Check sheet for the modelled part. Datum: model origin and axes. Units: mm. A direction names the side the tool comes from. Round coordinates to 2 decimals unless told otherwise and drop trailing zeros. Write each loop counter-clockwise with the first axis right and the second up, starting at its lowest first coordinate (ties: lowest second). Pieces come first, ordered by that corner, then holes.
Item 1: Release check for a two-part mould opening along Y. For faces 1 (the flat face through (-26, -13, 2)), 2 (the flat face through (-22, -13, 0.99)), 3 (the flat face through (-25, -35.09, 9)) record: +Y half, -Y half, draft (parallel to the pull), parting line (faces both ways), or undercut.
Item 2: Cross-section at B-B on x = -19. Enter the section's corners in (y, z).
Item 3: Cross-section at C-C on z = 18.5. Enter the section's corners in (x, y).
Item 4: Tool access check on faces 4 (the cylindrical face through (-19.49, 3.689, 3.287)), 5 (the cylindrical face through (-13.079, -2.82, 5.062)), 6 (the cylindrical face through (-19.438, -22.617, 3.561)), 7 (the flat face through (-9.914, -30, 10)), 8 (the cylindrical face through (-9.023, -30.055, 6.325)). Record the directions out of +Z, -Z, +X, -X, +Y, -Y that give a thin tool (end or side, any length) a straight path to the whole face; none if there is none.
Item 5: Cross-section at D-D on y = -1.5. Enter the section's corners in (x, z).
Item 6: Material ranges on line 1 (Y direction, x = -32, z = 17.25); line 2 (Y direction, x = -18.9, z = 6); line 3 (X direction, y = 1.5, z = 2.5), recorded low to high.
Item 7: Cross-section at A-A on y = 3. Enter the section's corners in (x, z), plus the area to 3 significant figures.
Item 8: Go/stop test with flat-tipped pins: pin 1 Ø1.6 at (y, z) = (2.5, 5.5) entering from -X; pin 2 Ø10 at (y, z) = (-30, 13.5) entering from +X; pin 3 Ø5 at (y, z) = (2.41, 6) entering from -X; pin 4 Ø8.5 at (x, y) = (-27.5, -15) entering from +Z. Record where each tip stops, or that it passes through.
from build123d import *

# Parameters (mm, degrees)
CROQUIS1_W               = 25
CROQUIS1_H               = 44
SALIENTE_EXTRUIR1_DEPTH  = 20
CROQUIS2_W               = 11.3
CROQUIS2_H               = 40.4
CORTAR_EXTRUIR1_DEPTH    = 18
CROQUIS3_W               = 10.7
CROQUIS3_H               = 44
CORTAR_EXTRUIR2_DEPTH    = 12
CORTAR_EXTRUIR3_START    = -25
CROQUIS4_R               = 1.6
CORTAR_EXTRUIR3_DEPTH    = 25
CROQUIS5_R               = 3
CORTAR_EXTRUIR4_DEPTH    = 17
CROQUIS7_W               = 10.7
CROQUIS7_H               = 2.131966011
SALIENTE_EXTRUIR2_DEPTH  = 12
CROQUIS9_W               = 11.3
CROQUIS9_H               = 12.16552506
SALIENTE_EXTRUIR3_DEPTH  = 2
SALIENTE_EXTRUIR4_DEPTH  = 2
CORTAR_EXTRUIR10_START   = -25
CROQUIS12_W              = 0.99
CROQUIS12_H              = 44
CORTAR_EXTRUIR10_DEPTH   = 25
CROQUIS13_W              = 8
CROQUIS13_H              = 44
CORTAR_EXTRUIR11_DEPTH   = 11.7
SALIENTE_EXTRUIR5_DEPTH  = 11.7
CROQUIS15_W              = 10.763613753
CROQUIS15_H              = 40.736067978
CORTAR_EXTRUIR12_DEPTH   = 4
CROQUIS16_R              = 1.5
SALIENTE_EXTRUIR6_DEPTH  = 1.2
CORTAR_EXTRUIR13_START   = -44
CORTAR_EXTRUIR13_DEPTH   = 44
CROQUIS18_W              = 0.936386247
CROQUIS18_H              = 40.568033989
CORTAR_EXTRUIR14_DEPTH   = 4
SALIENTE_EXTRUIR7_START  = -9.2
SALIENTE_EXTRUIR7_DEPTH  = 9.2
SALIENTE_EXTRUIR8_START  = -12.9
CROQUIS20_W              = 4
CROQUIS20_H              = 0.236067978
CROQUIS20_H_2            = 0.25
SALIENTE_EXTRUIR8_DEPTH  = 12.9
CROQUIS21_W              = 4
CROQUIS21_H              = 6.401046148
CROQUIS21_H_2            = 6.387114126
SALIENTE_EXTRUIR9_DEPTH  = 1.5
SALIENTE_EXTRUIR10_DEPTH = 0.4


with BuildPart() as part:
    # Croquis1 → Saliente-Extruir1 (new body)
    with BuildSketch(Plane.XY):
        with Locations((-22.114132301, -13.090425532)):
            Rectangle(CROQUIS1_W, CROQUIS1_H)
    extrude(amount=SALIENTE_EXTRUIR1_DEPTH)

    # Croquis2 → Cortar-Extruir1 (cut)
    with BuildSketch(Plane.XY.offset(20)):
        with Locations((-26.964132301, -13.090425532)):
            Rectangle(CROQUIS2_W, CROQUIS2_H)
    extrude(amount=-CORTAR_EXTRUIR1_DEPTH, mode=Mode.SUBTRACT)

    # Croquis3 → Cortar-Extruir2 (cut)
    with BuildSketch(Plane.XY.offset(20)):
        with Locations((-14.964132301, -13.090425532)):
            Rectangle(CROQUIS3_W, CROQUIS3_H)
    extrude(amount=-CORTAR_EXTRUIR2_DEPTH, mode=Mode.SUBTRACT)

    # Croquis4 → Cortar-Extruir3 (cut)
    with BuildSketch(Plane.ZY.offset(34.614132301).offset(CORTAR_EXTRUIR3_START)):
        with Locations((6, 2.409574468)):
            Circle(CROQUIS4_R)
        with Locations((6, -28.590425532)):
            Circle(CROQUIS4_R)
        with BuildLine():
            Line((20, 5.909574468), (20, -32.090425532))
            ThreePointArc((20, -32.090425532), (1, -13.090425532), (20, 5.909574468))
        make_face()
    extrude(amount=CORTAR_EXTRUIR3_DEPTH, mode=Mode.SUBTRACT)

    # Croquis5 → Cortar-Extruir4 (cut)
    with BuildSketch(Plane.ZY.offset(34.614132301)):
        with Locations((6, 2.409574468)):
            Circle(CROQUIS5_R)
        with Locations((6, -28.590425532)):
            Circle(CROQUIS5_R)
    extrude(amount=-CORTAR_EXTRUIR4_DEPTH, mode=Mode.SUBTRACT)

    # Croquis7 → Saliente-Extruir2 (add)
    with BuildSketch(Plane.XY.offset(8)):
        with Locations((-14.964132301, -34.024442527)):
            Rectangle(CROQUIS7_W, CROQUIS7_H)
        with Locations((-14.964132301, 7.843591463)):
            Rectangle(CROQUIS7_W, CROQUIS7_H)
    extrude(amount=SALIENTE_EXTRUIR2_DEPTH)

    # Croquis9 → Saliente-Extruir3 (add)
    with BuildSketch(Plane.XY.offset(2)):
        with Locations((-26.964132301, -13.090425532)):
            Rectangle(CROQUIS9_W, CROQUIS9_H)
    extrude(amount=-SALIENTE_EXTRUIR3_DEPTH)

    # Croquis11 → Saliente-Extruir4 (add)
    with BuildSketch(Plane.ZY.offset(32.614132301)):
        with BuildLine():
            Line((2, -7.007663002), (2, -19.173188062))
            ThreePointArc((2, -19.173188062), (1, -13.090425532), (2, -7.007663002))
        make_face()
    extrude(amount=SALIENTE_EXTRUIR4_DEPTH)

    # Croquis12 → Cortar-Extruir10 (cut)
    with BuildSketch(Plane.ZY.offset(34.614132301).offset(CORTAR_EXTRUIR10_START)):
        with Locations((0.495, -13.090425532)):
            Rectangle(CROQUIS12_W, CROQUIS12_H)
    extrude(amount=CORTAR_EXTRUIR10_DEPTH, mode=Mode.SUBTRACT)

    # Croquis13 → Cortar-Extruir11 (cut)
    with BuildSketch(Plane(origin=(-9.614132301, 0, 0), x_dir=(0, 0, -1), z_dir=(1, 0, 0))):
        with Locations((-16, -13.090425532)):
            Rectangle(CROQUIS13_W, CROQUIS13_H)
    extrude(amount=-CORTAR_EXTRUIR11_DEPTH, mode=Mode.SUBTRACT)

    # Croquis14 → Saliente-Extruir5 (add)
    with BuildSketch(Plane(origin=(-21.314132301, 0, 0), x_dir=(0, 0, -1), z_dir=(1, 0, 0))):
        with BuildLine():
            Line((-2, -19.173188062), (-2, -7.007663002))
            ThreePointArc((-2, -7.007663002), (-1, -13.090425532), (-2, -19.173188062))
        make_face()
    extrude(amount=SALIENTE_EXTRUIR5_DEPTH)

    # Croquis15 → Cortar-Extruir12 (cut)
    with BuildSketch(Plane.XY.offset(12)):
        with Locations((-14.995939178, -13.090425532)):
            Rectangle(CROQUIS15_W, CROQUIS15_H)
    extrude(amount=-CORTAR_EXTRUIR12_DEPTH, mode=Mode.SUBTRACT)

    # Croquis16 → Saliente-Extruir6 (add)
    with BuildSketch(Plane(origin=(-9.614132301, 0, 0), x_dir=(0, 0, -1), z_dir=(1, 0, 0))):
        with BuildLine():
            Line((-8, -27.821345395), (-8, -33.458459521))
            Line((-8, -33.458459521), (-12, -33.458459521))
            Line((-12, -33.458459521), (-12, -35.090425532))
            Line((-12, -35.090425532), (-0.99, -35.090425532))
            Line((-0.99, -35.090425532), (-0.99, 8.909574468))
            Line((-0.99, 8.909574468), (-12, 8.909574468))
            Line((-12, 8.909574468), (-12, 7.277608457))
            Line((-12, 7.277608457), (-8, 7.277608457))
            Line((-8, 7.277608457), (-8, 1.640494331))
            ThreePointArc((-8, 1.640494331), (-4.389181434, -2.259804881), (-2, -7.007663002))
            Line((-2, -7.007663002), (-2, -19.173188062))
            ThreePointArc((-2, -19.173188062), (-4.389181434, -23.921046183), (-8, -27.821345395))
        make_face()
        with Locations((-6, -28.590425532)):
            Circle(CROQUIS16_R, mode=Mode.SUBTRACT)
        with Locations((-6, 2.409574468)):
            Circle(CROQUIS16_R, mode=Mode.SUBTRACT)
    extrude(amount=SALIENTE_EXTRUIR6_DEPTH)

    # Croquis17 → Cortar-Extruir13 (cut)
    with BuildSketch(Plane.XZ.offset(35.090425532).offset(CORTAR_EXTRUIR13_START)):
        Polygon((-21.314132301, 12), (-21.314132301, 20), (-27.964132301, 20), align=None)
    extrude(amount=CORTAR_EXTRUIR13_DEPTH, mode=Mode.SUBTRACT)

    # Croquis18 → Cortar-Extruir14 (cut)
    with BuildSketch(Plane.XY.offset(12)):
        with Locations((-20.845939178, -13.006408538)):
            Rectangle(CROQUIS18_W, CROQUIS18_H)
    extrude(amount=-CORTAR_EXTRUIR14_DEPTH, mode=Mode.SUBTRACT)

    # Croquis19 → Saliente-Extruir7 (add)
    with BuildSketch(Plane(origin=(-8.414132301, 0, 0), x_dir=(0, 0, -1), z_dir=(1, 0, 0)).offset(SALIENTE_EXTRUIR7_START)):
        with BuildLine():
            Line((-2, -19.173188062), (-2, -7.007663002))
            ThreePointArc((-2, -7.007663002), (-4.389181434, -2.259804881), (-8, 1.640494331))
            Line((-8, 1.640494331), (-8, 0.640494331))
            ThreePointArc((-8, 0.640494331), (-5.026875227, -2.874277954), (-3, -7.007663002))
            Line((-3, -7.007663002), (-3, -19.173188062))
            ThreePointArc((-3, -19.173188062), (-4.972698099, -23.341991528), (-8, -26.821345395))
            Line((-8, -26.821345395), (-8, -27.821345395))
            ThreePointArc((-8, -27.821345395), (-4.389181434, -23.921046183), (-2, -19.173188062))
        make_face()
    extrude(amount=SALIENTE_EXTRUIR7_DEPTH)

    # Croquis20 → Saliente-Extruir8 (add)
    with BuildSketch(Plane(origin=(-8.414132301, 0, 0), x_dir=(0, 0, -1), z_dir=(1, 0, 0)).offset(SALIENTE_EXTRUIR8_START)):
        with Locations((-10, -33.340425532)):
            Rectangle(CROQUIS20_W, CROQUIS20_H)
        with Locations((-10, 7.152608457)):
            Rectangle(CROQUIS20_W, CROQUIS20_H_2)
    extrude(amount=SALIENTE_EXTRUIR8_DEPTH)

    # Croquis21 → Saliente-Extruir9 (add)
    with BuildSketch(Plane(origin=(-8.414132301, 0, 0), x_dir=(0, 0, -1), z_dir=(1, 0, 0))):
        with Locations((-10, -30.021868469)):
            Rectangle(CROQUIS21_W, CROQUIS21_H)
        with Locations((-10, 3.834051394)):
            Rectangle(CROQUIS21_W, CROQUIS21_H_2)
    extrude(amount=-SALIENTE_EXTRUIR9_DEPTH)

    # Croquis22 → Saliente-Extruir10 (add)
    with BuildSketch(Plane.XY.offset(8)):
        Polygon((-9.914132301, 7.027608457), (-21.314132301, 7.027608457), (-21.314132301, 4.645642446), (-17.614132301, 4.645642446), (-17.614132301, 0.640494331), (-9.914132301, 0.640494331), align=None)
        Polygon((-9.914132301, -26.821345395), (-17.614132301, -26.821345395), (-17.614132301, -30.826493509), (-21.314132301, -30.826493509), (-21.314132301, -33.222391543), (-9.914132301, -33.222391543), align=None)
    extrude(amount=SALIENTE_EXTRUIR10_DEPTH)


solid = part.part
Response values:
1. face 1: undercut
1. face 2: draft
1. face 3: -Y half
2. outline: (-35.09, 0.99) - (8.91, 0.99) - (8.91, 12) - (7.03, 12) - (7.03, 8.4) - (4.65, 8.4) - (4.65, 8) arc R3 cw (long way) to (-0.58, 5.7) arc R19 cw to (-7.01, 2) - (-19.17, 2) arc R19 cw to (-25.61, 5.7) arc R3 cw (long way) to (-30.83, 8) - (-30.83, 8.4) - (-33.22, 8.4) - (-33.22, 12) - (-35.09, 12) - close
3. outline: (-34.61, -35.09) - (-26.72, -35.09) - (-26.72, -33.29) - (-32.61, -33.29) - (-32.61, -32.03) - (-34.61, -32.03) - close; (-34.61, 5.85) - (-32.61, 5.85) - (-32.61, 7.11) - (-26.72, 7.11) - (-26.72, 8.91) - (-34.61, 8.91) - close
4. face 4: -X
4. face 5: +Z, +X, -X
4. face 6: +Z, -X
4. face 7: +Z
4. face 8: +X, -X
5. outline: (-34.61, 0.99) - (-8.41, 0.99) - (-8.41, 6.02) - (-17.61, 6.02) - (-17.61, 4.94) - (-21.31, 4.94) - (-21.31, 2) - (-32.61, 2) - (-32.61, 4.94) - (-34.61, 4.94) - close
6. line 1: y = -35.09 to -33.29, 7.11 to 8.91
6. line 2: y = -35.09 to -31.59, 5.41 to 8.91
6. line 3: x = -34.61 to -32.61, -21.31 to -8.41
7. outline: (-34.61, 0.99) - (-8.41, 0.99) - (-8.41, 4.62) - (-9.61, 4.62) - (-9.61, 4.51) - (-17.61, 4.51) - (-17.61, 3.06) - (-21.31, 3.06) - (-21.31, 2) - (-32.61, 2) - (-32.61, 3.06) - (-34.61, 3.06) - close; (-34.61, 8.94) - (-32.61, 8.94) - (-32.61, 9.9) - (-34.61, 9.9) - close; (-17.61, 7.49) - (-9.61, 7.49) - (-9.61, 7.38) - (-8.41, 7.38) - (-8.41, 12) - (-9.91, 12) - (-9.91, 8.4) - (-17.61, 8.4) - close
7. area: 71.6 mm2
8. pin 1: passes through
8. pin 2: stops at x = -8.41
8. pin 3: stops at x = -17.61
8. pin 4: stops at z = 2
